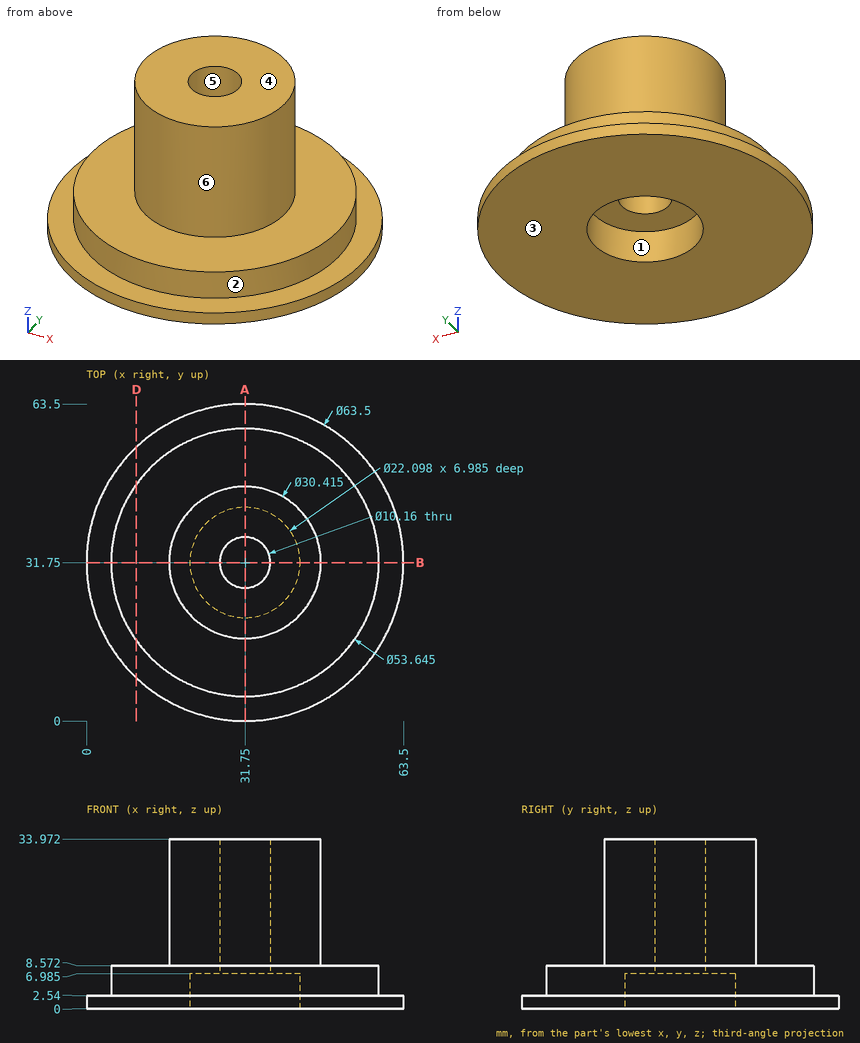
Can you work these out from the drawing? Everything is in mm from the part's minimum corner. A direction names the side the tool comes from. Coordinates: 2 decimals unless noted, no trailing zeros. Order: outer loops, then holes, each group sorted by start corner. A loop starts at its lowest first (then second) coordinate and runs counter-clockwise, first axis right, second up. Notation, with made-up numbers: M 52.25,-34 L 59.25,-34 A25 ccw 59.25,-8 Z; hole C 11,-30 d8. An arc over 180 degrees is marked long. Answer as CSV lines item,"result". Start each with the question number.
1. I need wall thicknesses on line 1 (Y direction, x = 31.75, z = 4); line 2 (Y direction, x = 32, z = 27.5) (1 decimal); line 3 (Z direction, x = 60, y = 41). Which ranges of each line are inside material? Lowest first, please. Write a range as [from, to].
2. I want a section at D-D, the plane x = 10. Write out the boundary of the cut face in (y, z).
3. We'd pull the mould along Y, two halves only. Please class the marked faces 4, 5 and 6: released by +Y, released by -Y, zero draft, split by the parting line, or undercut.
4. For pin 1 (1 mm diameter, centred on x = 33, y = 49, fed in from +Z); pin 2 (13 mm diameter, centred on x = 31.75, y = 31.75, fed in from -Z) (1 decimal); pin 3 (6 mm diameter, centred on x = 32.5, z = 8.5, fed in from +Y), each with a flat end and sliding along its axis, tell me the tip position at first contact or that it passes through.
5. I want a section at A-A, the plane x = 31.75. Write out the boundary of the cut face in (y, z) (1 decimal).
6. On a 3-axis mill with a long thin cutter (end or side, diameter ignored), from which of +Z, -Z, +X, -X, +Y, -Y can I reach the whole of each face in a straight line? I mean the marked faces 1, 2 and 3. Say none if no direction works.
Recorded:
1,line 1,"y = [4.93, 20.7], [42.8, 58.57]"
1,line 2,"y = [16.5, 26.7], [36.8, 47]"
1,line 3,"z = [0, 2.54]"
2,outline,"M 8.62,0 L 54.88,0 L 54.88,2.54 L 47.45,2.54 L 47.45,8.57 L 16.05,8.57 L 16.05,2.54 L 8.62,2.54 Z"
3,face 4,"zero draft"
3,face 5,"undercut"
3,face 6,"split by the parting line"
4,pin 1,"stops at z = 8.57"
4,pin 2,"stops at z = 7"
4,pin 3,"stops at y = 58.57"
5,outline,"M 0,0 L 20.7,0 L 20.7,7 L 26.7,7 L 26.7,34 L 16.5,34 L 16.5,8.6 L 4.9,8.6 L 4.9,2.5 L 0,2.5 Z; M 36.8,7 L 42.8,7 L 42.8,0 L 63.5,0 L 63.5,2.5 L 58.6,2.5 L 58.6,8.6 L 47,8.6 L 47,34 L 36.8,34 Z"
6,face 1,"-Z"
6,face 2,"+Z"
6,face 3,"-Z, +X, -X, +Y, -Y"
